Design review of the part built by this model. Coordinates are the model's own, in mm. A direction names the side the tool comes from. Round coordinates to 2 decimals unless told otherwise and drop trailing zeros. Loops run counter-clockwise (first coordinate to the right, second up) from the corner with the lowest first, then second, coordinate; pieces in that order, holes last. Notation, with made-up numbers: (15, 50.5) - (34, 50.5) arc R11 ccw to (34, 68.5) - close; hole circle Ø7 at (-32.5, 32.25). An arc over 180 degrees is marked (long way). Return JSON: item names as keys, results as strings. Group by question number.
from build123d import *

# Parameters (mm, degrees)
SKETCH_1_R          = 1.525
EXTRUDE_1_DEPTH     = 1.5
FILLET_1_R          = 2
CUT_EXTRUDE_1_DEPTH = 11.5
EXTRUDE_2_DEPTH     = 3
FILLET_2_R          = 2


with BuildPart() as part:
    # 草图1 → 凸台-拉伸1 (new, symmetric)
    with BuildSketch(Plane.XY):
        Polygon((-71.5, 19), (-40, 40), (40, 40), (71.5, 19), (71.5, -19), (-71.5, -19), align=None)
        with Locations((67.5, 15)):
            Circle(SKETCH_1_R, mode=Mode.SUBTRACT)
        with Locations((67.5, -15)):
            Circle(SKETCH_1_R, mode=Mode.SUBTRACT)
        with Locations((-67.5, -15)):
            Circle(SKETCH_1_R, mode=Mode.SUBTRACT)
        with Locations((-67.5, 15)):
            Circle(SKETCH_1_R, mode=Mode.SUBTRACT)
    extrude(amount=EXTRUDE_1_DEPTH, both=True)

    # 圆角1
    fillet_1_edges = [part.edges().sort_by_distance(p)[0] for p in [
        (71.5, 19, 0),
        (71.5, -19, 0),
        (-71.5, -19, 0),
        (-71.5, 19, 0),
        (-40, 40, 0),
        (40, 40, 0),
    ]]
    fillet(fillet_1_edges, radius=FILLET_1_R)

    # 草图2 → 切除-拉伸1 (cut, symmetric)
    with BuildSketch(Plane.XY.offset(1.5)):
        Polygon((-2.543149186, -14), (-24.770935731, 14.300111558), (-60.290463502, -14), align=None)
        Polygon((-40.058974879, 33.764632352), (-38.486121811, 35), (-63.5, 18.324081208), (-63.5, -11.442808319), (-27.241730885, 17.445893903), align=None)
        Polygon((-5.209536498, 35), (-35.942972625, 35), (-24.113223205, 19.938526038), align=None)
        Polygon((-2, 32.442808319), (-21.642428051, 16.792743692), (-2, -8.215725055), align=None)
        Polygon((21.642428051, 16.792743692), (2, 32.442808319), (2, -8.215725055), align=None)
        Polygon((35.942972625, 35), (5.209536498, 35), (24.113223205, 19.938526038), align=None)
        Polygon((63.5, 18.324081208), (38.486121811, 35), (40.058974879, 33.764632352), (27.241730885, 17.445893903), (63.5, -11.442808319), align=None)
        Polygon((24.770935731, 14.300111558), (2.543149186, -14), (60.290463502, -14), align=None)
    extrude(amount=CUT_EXTRUDE_1_DEPTH, both=True, mode=Mode.SUBTRACT)

    # 草图3 → 凸台-拉伸2 (add)
    with BuildSketch(Plane.XY.offset(1.5)):
        Polygon((40.058974879, 33.764632352), (40.676658703, 34.551058886), (38.486121811, 35), align=None)
    extrude_2 = extrude(amount=-EXTRUDE_2_DEPTH)

    # 镜向1: 凸台-拉伸2 across plane
    add(extrude_2.mirror(Plane(origin=(0, 0, 0), x_dir=(0, 0, 1), z_dir=(1, 0, 0))))

    # 圆角2
    fillet_2_edges = [part.edges().sort_by_distance(p)[0] for p in [
        (2, 32.442808319, 0),
        (21.642428051, 16.792743692, 0),
        (2, -8.215725055, 0),
        (-21.642428051, 16.792743692, 0),
        (-2, 32.442808319, 0),
        (-2, -8.215725055, 0),
        (-63.5, -11.442808319, 0),
        (-63.5, 18.324081208, 0),
        (-27.241730885, 17.445893903, 0),
        (-24.113223205, 19.938526038, 0),
        (-35.942972625, 35, 0),
        (-5.209536498, 35, 0),
        (24.770935731, 14.300111558, 0),
        (60.290463502, -14, 0),
        (2.543149186, -14, 0),
        (5.209536498, 35, 0),
        (35.942972625, 35, 0),
        (24.113223205, 19.938526038, 0),
        (27.241730885, 17.445893903, 0),
        (63.5, 18.324081208, 0),
        (63.5, -11.442808319, 0),
        (-60.290463502, -14, 0),
        (-24.770935731, 14.300111558, 0),
        (-2.543149186, -14, 0),
        (40.155270293, 33.887234346, 0),
        (-40.155270293, 33.887234346, 0),
    ]]
    fillet(fillet_2_edges, radius=FILLET_2_R)


solid = part.part
Q1. For line 1 (Y direction, x = 28, z = 0.85); line 2 (Y direction, x = -67.5, z = 0.1) (3 decimals); line 3 (Y direction, x = 20, z = -0.35), list the stretches that pass through material, from the lowest coordinate up.
Q2. Tool access review of faces 4 (the flat face through (71.5, 1, 0)), 5 (the flat face through (30, -14, 0)): name each direction out of +Z, -Z, +X, -X, +Y, -Y from which nothing blocks a thin tool from reaching the whole face with its end or side.
Q3. Add section C-C, the plane x = -18. State the section outline as (y, z) points.
Q4. Add section A-A, the plane x = -67.5. State the section outline as (y, z) points (3 decimals), plus the area to 3 significant figures.
Q5. Add section B-B, the plane y = 4. State the section outline as (x, z) points, plus the area to 3 significant figures.
Q6. Add section D-D, the plane z = -0.55. Give the number of separate pieces and of enclosed holes in the cut face, plus the area to 3 significant figures.
Q7. Draft analysis for pull direction Y (two halves, no side actions). For faces 1 (the flat face through (-55.767, 29.488, 0.021)), 2 (the cylindrical face through (-62.4, -9.08, -0.02)), 3 (the flat face through (1, 11, -1.5)), state which applies: pulls with the +Y half, pulls with the -Y half, needs draft (parallel to the pull), parting line crosses it, or undercut.
Q8. Insertion check: pin 1 Ø1 at (y, z) = (22.5, -1) entering from -X. The pin has a flat end and moves straight along its axis. Give the tip position at first contact, or say it passes through.
Evaluation:
{
 "1": {"line 1": "-19 to -14, 11.73 to 24.89, 35 to 40", "line 2": "-19 to -16.525, -13.475 to 13.475, 16.525 to 21.667", "line 3": "-19 to -14, 8.23 to 14.7, 18.1 to 23.22, 35 to 40"},
 "2": {"face 4": "+Z, -Z, +X, +Y, -Y", "face 5": "+Z, -Z"},
 "3": {"outline": "(-19, -1.5) - (-14, -1.5) - (-14, 1.5) - (-19, 1.5) - close; (5.68, -1.5) - (12.16, -1.5) - (12.16, 1.5) - (5.68, 1.5) - close; (19.69, -1.5) - (24.81, -1.5) - (24.81, 1.5) - (19.69, 1.5) - close; (35, -1.5) - (40, -1.5) - (40, 1.5) - (35, 1.5) - close"},
 "4": {"outline": "(-19, -1.5) - (-16.525, -1.5) - (-16.525, 1.5) - (-19, 1.5) - close; (-13.475, -1.5) - (13.475, -1.5) - (13.475, 1.5) - (-13.475, 1.5) - close; (16.525, -1.5) - (21.667, -1.5) - (21.667, 1.5) - (16.525, 1.5) - close", "area": "104 mm²"},
 "5": {"outline": "(-71.5, -1.5) - (-63.5, -1.5) - (-63.5, 1.5) - (-71.5, 1.5) - close; (-44.12, -1.5) - (-37.7, -1.5) - (-37.7, 1.5) - (-44.12, 1.5) - close; (-16.68, -1.5) - (-11.59, -1.5) - (-11.59, 1.5) - (-16.68, 1.5) - close; (-2, -1.5) - (2, -1.5) - (2, 1.5) - (-2, 1.5) - close; (11.59, -1.5) - (16.68, -1.5) - (16.68, 1.5) - (11.59, 1.5) - close; (37.7, -1.5) - (44.12, -1.5) - (44.12, 1.5) - (37.7, 1.5) - close; (63.5, -1.5) - (71.5, -1.5) - (71.5, 1.5) - (63.5, 1.5) - close", "area": "129 mm²"},
 "6": {"separate pieces": "1", "enclosed holes": "12", "area": "3,260 mm²"},
 "7": {"face 1": "pulls with the +Y half", "face 2": "undercut", "face 3": "needs draft"},
 "8": {"pin 1": "x = -67"}
}
